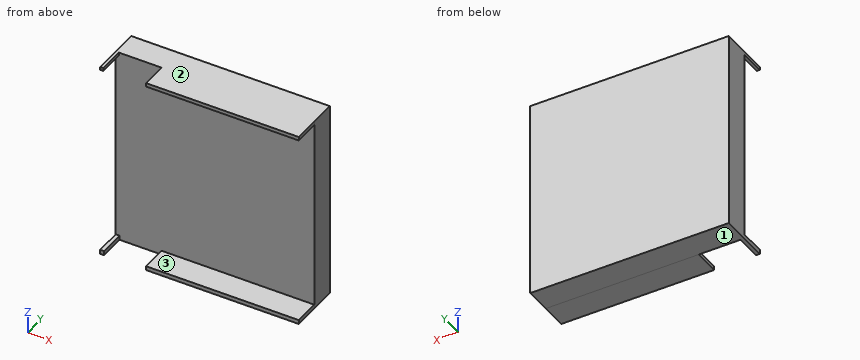
```python
from build123d import *

# Parameters (mm, degrees)
F0_W     = 305
F0_H     = 306.783354
F1_DEPTH = 40
F2_W     = 4.656996
F2_H     = 4.847504
F3_DEPTH = 40
F4_W     = 234.520369
F4_H     = 5.697318
F5_DEPTH = 40
F6_W     = 5.924162
F6_H     = 6.802148
F7_DEPTH = 40
F8_W     = 234.898739
F8_H     = 6.330257
F9_DEPTH = 40


with BuildPart() as f1:
    # F0 (on Front) → F1 (new body)
    with BuildSketch(Plane.XZ):
        with Locations((152.5, 153.391677)):
            Rectangle(F0_W, F0_H)
    extrude(amount=F1_DEPTH)

    # F2 (on face) → F3 (join)
    with BuildSketch(Plane.XZ.offset(40)):
        with Locations((2.328498, 304.359602)):
            Rectangle(F2_W, F2_H)
    extrude(amount=F3_DEPTH)

    # F4 (on face) → F5 (join)
    with BuildSketch(Plane.XZ.offset(40)):
        with Locations((187.739815, 303.934695)):
            Rectangle(F4_W, F4_H)
    extrude(amount=F5_DEPTH)

    # F6 (on face) → F7 (join)
    with BuildSketch(Plane.XZ.offset(40)):
        with Locations((2.962081, 3.401074)):
            Rectangle(F6_W, F6_H)
    extrude(amount=F7_DEPTH)

    # F8 (on face) → F9 (join)
    with BuildSketch(Plane.XZ.offset(40)):
        with Locations((187.550631, 3.165128)):
            Rectangle(F8_W, F8_H)
    extrude(amount=F9_DEPTH)


solid = f1.part
```
Check sheet for the modelled part. Datum: model origin and axes. Units: mm. Face numbers are marked on the shaded views. Give positions to 0.01 mm unless a question says otherwise; leave off trailing zeros. Order: outer loops, then holes, each group sorted by start corner. A loop starts at its lowest first (then second) coordinate and runs counter-clockwise, first axis right, second up. Notation, with made-up numbers: (87.25, 55) -> (129.25, 55) arc R28 ccw to (129.25, 86) -> close; hole circle Ø1 at (-4, 25). An arc over 180 degrees is marked (long way). Use CSV: the item, a comma, the result in double quotes. Start each with the question number.
1) Sectioned sample at D-D, the plane x = 25. Record the boundary of the cut face in (y, z), plus the area to 3 significant figures.
2) Sectioned sample at C-C, the plane z = 164. Record the boundary of the cut face in (x, y), plus the area to 3 significant figures.
3) Material ranges on line 1 (Z direction, x = 150, y = -77); line 2 (Y direction, x = 30, z = 67), recorded low to high. Write a range as from..to.
4) Sectioned sample at A-A, the plane y = -73.5. Record the boundary of the cut face in (x, z), plus the area to 3 significant figures.
5) Go/stop test with a flat-tipped pin: P1, Ø7, axis at y = -50.5, z = 3.5, coming from the -X side. Record where the tip stops, or that it passes through.
6) Mould release check, pull along Z, two halves, no side actions. Record for the marked faces 1, 2 and 3: released by +Z, released by -Z, zero draft, split by the parting line, or undercut.
7) Sectioned sample at B-B, the plane x = 173.5. Record the boundary of the cut face in (y, z), plus the area to 3 significant figures.
Recorded:
1,outline,"(-40, 0) -> (0, 0) -> (0, 306.78) -> (-40, 306.78) -> close"
1,area,"12,300 mm2"
2,outline,"(0, -40) -> (305, -40) -> (305, 0) -> (0, 0) -> close"
2,area,"12,200 mm2"
3,line 1,"0..6.33, 301.09..306.78"
3,line 2,"-40..0"
4,outline,"(0, 0) -> (5.92, 0) -> (5.92, 6.8) -> (0, 6.8) -> close; (0, 301.94) -> (4.66, 301.94) -> (4.66, 306.78) -> (0, 306.78) -> close; (70.1, 0) -> (305, 0) -> (305, 6.33) -> (70.1, 6.33) -> close; (70.48, 301.09) -> (305, 301.09) -> (305, 306.78) -> (70.48, 306.78) -> close"
4,area,"2,890 mm2"
5,P1,"x = 0"
6,face 1,"released by -Z"
6,face 2,"released by +Z"
6,face 3,"undercut"
7,outline,"(-80, 0) -> (0, 0) -> (0, 306.78) -> (-80, 306.78) -> (-80, 301.09) -> (-40, 301.09) -> (-40, 6.33) -> (-80, 6.33) -> close"
7,area,"12,800 mm2"
